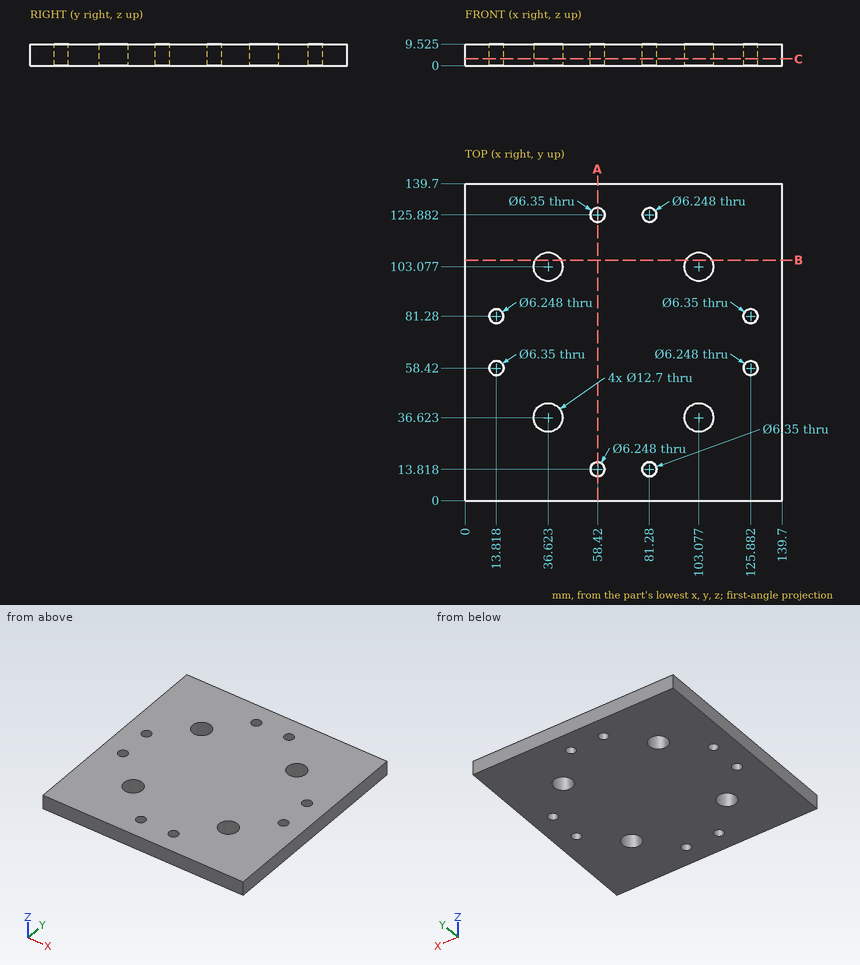
Can you work these out from the drawing? Everything is in mm from the part's minimum corner. Give positions to 0.01 mm unless a question says otherwise; leave off trailing zeros. Write each loop counter-clockwise with the first axis right and the second up, starting at its lowest first coordinate (ties: lowest second). Pieces come first, ordered by that corner, then holes. Notation, with made-up numbers: M 75,-11 L 99,-11 A19 cw 99,21 Z; hole C -21.5,62 d10. An arc over 180 degrees is marked long. Answer in a Markdown table with one row per item. Add a question column.
Item 1: Imagine slicing it at C-C, the plane z = 3. State how many separate pieces and enclosed holes the cut face has, plus the area to 3 significant figures.
Item 2: Imagine slicing it at A-A, the plane x = 58.42. Write out the boundary of the cut face in (y, z) (1 decimal).
Item 3: Please list where these lines run through material, in increasing order: L1, parallel to Y at x = 125.5, z = 3.5; L2, parallel to X at y = 80, z = 6.5; L3, parallel to Y at x = 100, z = 5.5.
Item 4: Imagine slicing it at B-B, the plane y = 106. Write out the boundary of the cut face in (x, z) (1 decimal), plus the area to 3 significant figures.
Evaluation:
| question | item | result |
|---|---|---|
| 1 | separate pieces | 1 |
| 1 | enclosed holes | 12 |
| 1 | area | 18,800 mm² |
| 2 | outline | M 0,0 L 10.7,0 L 10.7,9.5 L 0,9.5 Z; M 16.9,0 L 122.7,0 L 122.7,9.5 L 16.9,9.5 Z; M 129.1,0 L 139.7,0 L 139.7,9.5 L 129.1,9.5 Z |
| 3 | L1 | y = 0 to 55.32, 61.52 to 78.13, 84.43 to 139.7 |
| 3 | L2 | x = 0 to 10.97, 16.67 to 122.98, 128.79 to 139.7 |
| 3 | L3 | y = 0 to 31.07, 42.18 to 97.52, 108.63 to 139.7 |
| 4 | outline | M 0,0 L 31,0 L 31,9.5 L 0,9.5 Z; M 42.3,0 L 97.4,0 L 97.4,9.5 L 42.3,9.5 Z; M 108.7,0 L 139.7,0 L 139.7,9.5 L 108.7,9.5 Z |
| 4 | area | 1,120 mm² |
